```python
from build123d import *

# Parameters (mm, degrees)
BOSS_EXTRUDE1_DEPTH = 55
SKETCH2_W           = 12
SKETCH2_H           = 4.5
SKETCH2_W_2         = 11.8
SKETCH2_H_2         = 4.3
BOSS_EXTRUDE2_DEPTH = 12.5
SKETCH3_W           = 11.8
SKETCH3_H           = 1.5
BOSS_EXTRUDE3_DEPTH = 12.4
CUT_EXTRUDE1_DEPTH  = 0.5
SKETCH6_W           = 10.75
SKETCH6_H           = 9
CUT_EXTRUDE2_DEPTH  = 3
SKETCH7_W           = 5.5
SKETCH7_H           = 2.3
BOSS_EXTRUDE4_DEPTH = 0.1
SKETCH8_R           = 0.3
BOSS_EXTRUDE5_DEPTH = 6
LPATTERN1_COUNT     = 3
LPATTERN1_PITCH     = 2.9
SKETCH9_W           = 15.5
SKETCH9_H           = 3.5
CUT_EXTRUDE3_DEPTH  = 2
SKETCH10_R          = 0.3
BOSS_EXTRUDE6_DEPTH = 6
LPATTERN2_COUNT     = 6
LPATTERN2_PITCH     = 2.5
FILLET1_R           = 1.25


with BuildPart() as part:
    # Sketch1 → Boss-Extrude1 (new body)
    with BuildSketch(Plane.XY):
        Polygon((-12.5, 0), (-12, -6.2), (12, -6.2), (12.5, 0), (12.5, 5.5), (-12.5, 5.5), align=None)
    extrude(amount=-BOSS_EXTRUDE1_DEPTH)

    # Sketch2 → Boss-Extrude2 (add)
    with BuildSketch(Plane.XY):
        Rectangle(SKETCH2_W, SKETCH2_H)
        Rectangle(SKETCH2_W_2, SKETCH2_H_2, mode=Mode.SUBTRACT)
    extrude(amount=BOSS_EXTRUDE2_DEPTH)

    # Sketch3 → Boss-Extrude3 (add)
    with BuildSketch(Plane.XY):
        with Locations((0, -1.4)):
            Rectangle(SKETCH3_W, SKETCH3_H)
    extrude(amount=BOSS_EXTRUDE3_DEPTH)

    # Sketch4 → Cut-Extrude1 (cut)
    with BuildSketch(Plane(origin=(0, 2.25, 0), x_dir=(1, 0, 0), z_dir=(0, 1, 0))):
        with BuildLine():
            Line((-4.25, -5.3), (-1.95, -5.3))
            ThreePointArc((-1.95, -5.3), (-1.808578644, -5.358578644), (-1.75, -5.5))
            Line((-1.75, -5.5), (-1.75, -7.3))
            ThreePointArc((-1.75, -7.3), (-1.808578644, -7.441421356), (-1.95, -7.5))
            Line((-1.95, -7.5), (-4.25, -7.5))
            ThreePointArc((-4.25, -7.5), (-4.391421356, -7.441421356), (-4.45, -7.3))
            Line((-4.45, -7.3), (-4.45, -5.5))
            ThreePointArc((-4.45, -5.5), (-4.391421356, -5.358578644), (-4.25, -5.3))
        make_face()
        with BuildLine():
            Line((1.95, -5.3), (4.25, -5.3))
            ThreePointArc((4.25, -5.3), (4.391421356, -5.358578644), (4.45, -5.5))
            Line((4.45, -5.5), (4.45, -7.3))
            ThreePointArc((4.45, -7.3), (4.391421356, -7.441421356), (4.25, -7.5))
            Line((4.25, -7.5), (1.95, -7.5))
            ThreePointArc((1.95, -7.5), (1.808578644, -7.441421356), (1.75, -7.3))
            Line((1.75, -7.3), (1.75, -5.5))
            ThreePointArc((1.75, -5.5), (1.808578644, -5.358578644), (1.95, -5.3))
        make_face()
    extrude(amount=-CUT_EXTRUDE1_DEPTH, mode=Mode.SUBTRACT)

    # Sketch6 → Cut-Extrude2 (cut)
    with BuildSketch(Plane(origin=(0, 5.5, 0), x_dir=(1, 0, 0), z_dir=(0, 1, 0))):
        with Locations((-7.125, 18)):
            Rectangle(SKETCH6_W, SKETCH6_H)
    extrude(amount=-CUT_EXTRUDE2_DEPTH, mode=Mode.SUBTRACT)

    # Sketch7 → Boss-Extrude4 (add)
    with BuildSketch(Plane(origin=(0, 2.5, 0), x_dir=(1, 0, 0), z_dir=(0, 1, 0))):
        with Locations((-6.75, 15.15)):
            Rectangle(SKETCH7_W, SKETCH7_H)
    boss_extrude4 = extrude(amount=BOSS_EXTRUDE4_DEPTH)

    # Sketch8 → Boss-Extrude5 (add)
    with BuildSketch(Plane(origin=(0, 2.6, 0), x_dir=(1, 0, 0), z_dir=(0, 1, 0))):
        with Locations(Location((-8, 15.15, 0), (0, 0, 180))):
            Circle(SKETCH8_R)
        with Locations(Location((-5.5, 15.15, 0), (0, 0, 180))):
            Circle(SKETCH8_R)
    boss_extrude5 = extrude(amount=BOSS_EXTRUDE5_DEPTH)

    # LPattern1: Boss-Extrude4, Boss-Extrude5 ×3
    with Locations(*[(0, 0, -i * LPATTERN1_PITCH) for i in range(1, LPATTERN1_COUNT)]):
        add(boss_extrude4)
        add(boss_extrude5)

    # Sketch9 → Cut-Extrude3 (cut)
    with BuildSketch(Plane(origin=(0, 0, -55), x_dir=(-1, 0, 0), z_dir=(0, 0, -1))):
        with Locations((0, 1.75)):
            Rectangle(SKETCH9_W, SKETCH9_H)
    extrude(amount=-CUT_EXTRUDE3_DEPTH, mode=Mode.SUBTRACT)

    # Sketch10 → Boss-Extrude6 (add)
    with BuildSketch(Plane(origin=(0, 0, -53), x_dir=(-1, 0, 0), z_dir=(0, 0, -1))):
        with Locations((-6.25, 1.75)):
            Circle(SKETCH10_R)
    boss_extrude6 = extrude(amount=BOSS_EXTRUDE6_DEPTH)

    # LPattern2: Boss-Extrude6 ×6
    with Locations(*[(-i * LPATTERN2_PITCH, 0, 0) for i in range(1, LPATTERN2_COUNT)]):
        add(boss_extrude6)

    # Fillet1
    # the kernel refuses this fillet: 1.25 mm, written as the material it takes off along each edge
    with BuildSketch(Plane(origin=(11.25, 4.25, -1.25), x_dir=(0, 0, 1), z_dir=(1, 0, 0))) as fillet1_piece_1_section:
        Polygon((0, 0), (FILLET1_R * 1.02, 0), (FILLET1_R * 1.02, -FILLET1_R * 1.02), (0, -FILLET1_R * 1.02), align=None)
    fillet1_piece_1 = extrude(amount=FILLET1_R * 1.02, mode=Mode.PRIVATE)
    fillet1_piece_1 = fillet1_piece_1 - Plane(origin=(11.25, 4.25, -1.25), x_dir=(0, -0.7071067811865475, -0.7071067811865475), z_dir=(1, 0, 0)) * Sphere(FILLET1_R, mode=Mode.PRIVATE)
    add(fillet1_piece_1, mode=Mode.SUBTRACT)
    with BuildSketch(Plane(origin=(-11.25, 4.25, -1.25), x_dir=(0, 0, 1), z_dir=(-1, 0, 0))) as fillet1_piece_2_section:
        Polygon((0, 0), (FILLET1_R * 1.02, 0), (FILLET1_R * 1.02, FILLET1_R * 1.02), (0, FILLET1_R * 1.02), align=None)
    fillet1_piece_2 = extrude(amount=FILLET1_R * 1.02, mode=Mode.PRIVATE)
    fillet1_piece_2 = fillet1_piece_2 - Plane(origin=(-11.25, 4.25, -1.25), x_dir=(0, -0.7071067811865475, -0.7071067811865475), z_dir=(-1, 0, 0)) * Sphere(FILLET1_R, mode=Mode.PRIVATE)
    add(fillet1_piece_2, mode=Mode.SUBTRACT)
    with BuildSketch(Plane(origin=(-11.25, 4.25, -53.75), x_dir=(0, 0, -1), z_dir=(-1, 0, 0))) as fillet1_piece_3_section:
        Polygon((0, 0), (FILLET1_R * 1.02, 0), (FILLET1_R * 1.02, -FILLET1_R * 1.02), (0, -FILLET1_R * 1.02), align=None)
    fillet1_piece_3 = extrude(amount=FILLET1_R * 1.02, mode=Mode.PRIVATE)
    fillet1_piece_3 = fillet1_piece_3 - Plane(origin=(-11.25, 4.25, -53.75), x_dir=(0, -0.7071067811865475, 0.7071067811865475), z_dir=(-1, 0, 0)) * Sphere(FILLET1_R, mode=Mode.PRIVATE)
    add(fillet1_piece_3, mode=Mode.SUBTRACT)
    with BuildSketch(Plane(origin=(11.25, 4.25, -53.75), x_dir=(0, 0, -1), z_dir=(1, 0, 0))) as fillet1_piece_4_section:
        Polygon((0, 0), (FILLET1_R * 1.02, 0), (FILLET1_R * 1.02, FILLET1_R * 1.02), (0, FILLET1_R * 1.02), align=None)
    fillet1_piece_4 = extrude(amount=FILLET1_R * 1.02, mode=Mode.PRIVATE)
    fillet1_piece_4 = fillet1_piece_4 - Plane(origin=(11.25, 4.25, -53.75), x_dir=(0, -0.7071067811865475, 0.7071067811865475), z_dir=(1, 0, 0)) * Sphere(FILLET1_R, mode=Mode.PRIVATE)
    add(fillet1_piece_4, mode=Mode.SUBTRACT)
    with BuildSketch(Plane(origin=(-19.5, -6.2, 0), x_dir=(0, 0, -1), z_dir=(1, 0, 0))) as fillet1_piece_5:
        with BuildLine():
            CenterArc((FILLET1_R, FILLET1_R), FILLET1_R, 180, 90)
            Line((0, FILLET1_R), (-FILLET1_R * 0.02, FILLET1_R))
            Line((-FILLET1_R * 0.02, FILLET1_R), (-FILLET1_R * 0.02, -FILLET1_R * 0.02))
            Line((-FILLET1_R * 0.02, -FILLET1_R * 0.02), (FILLET1_R, -FILLET1_R * 0.02))
            Line((FILLET1_R, -FILLET1_R * 0.02), (FILLET1_R, 0))
        make_face()
    extrude(amount=39, mode=Mode.SUBTRACT)
    with BuildSketch(Plane(origin=(11.25, 5.5, 0), x_dir=(0, -1, 0), z_dir=(-1, 0, 0))) as fillet1_piece_6:
        with BuildLine():
            CenterArc((FILLET1_R, -FILLET1_R), FILLET1_R, 90, 90)
            Line((0, -FILLET1_R), (-FILLET1_R * 0.02, -FILLET1_R))
            Line((-FILLET1_R * 0.02, -FILLET1_R), (-FILLET1_R * 0.02, FILLET1_R * 0.02))
            Line((-FILLET1_R * 0.02, FILLET1_R * 0.02), (FILLET1_R, FILLET1_R * 0.02))
            Line((FILLET1_R, FILLET1_R * 0.02), (FILLET1_R, 0))
        make_face()
    extrude(amount=22.5, mode=Mode.SUBTRACT)
    with BuildSketch(Plane(origin=(-12.5, 5.5, -1.25), x_dir=(0, -1, 0), z_dir=(0, 0, -1))) as fillet1_piece_7:
        with BuildLine():
            CenterArc((FILLET1_R, -FILLET1_R), FILLET1_R, 90, 90)
            Line((0, -FILLET1_R), (-FILLET1_R * 0.02, -FILLET1_R))
            Line((-FILLET1_R * 0.02, -FILLET1_R), (-FILLET1_R * 0.02, FILLET1_R * 0.02))
            Line((-FILLET1_R * 0.02, FILLET1_R * 0.02), (FILLET1_R, FILLET1_R * 0.02))
            Line((FILLET1_R, FILLET1_R * 0.02), (FILLET1_R, 0))
        make_face()
    extrude(amount=19.75, mode=Mode.SUBTRACT)
    with BuildSketch(Plane(origin=(-12.5, 5.5, -15), x_dir=(0, -1, 0), z_dir=(0, 0, -1))) as fillet1_piece_8:
        with BuildLine():
            CenterArc((FILLET1_R, -FILLET1_R), FILLET1_R, 90, 90)
            Line((0, -FILLET1_R), (-FILLET1_R * 0.02, -FILLET1_R))
            Line((-FILLET1_R * 0.02, -FILLET1_R), (-FILLET1_R * 0.02, FILLET1_R * 0.02))
            Line((-FILLET1_R * 0.02, FILLET1_R * 0.02), (FILLET1_R, FILLET1_R * 0.02))
            Line((FILLET1_R, FILLET1_R * 0.02), (FILLET1_R, 0))
        make_face()
    extrude(amount=38.75, mode=Mode.SUBTRACT)
    with BuildSketch(Plane(origin=(-12, -6.2, 6.919510423), x_dir=(-0.08038418992031013, 0.9967639550118451, 0), z_dir=(0, 0, -1)), Plane(origin=(12, -6.2, 6.919510423), x_dir=(-1, 0, 0), z_dir=(0, 0, -1))) as fillet1_piece_9:
        with BuildLine():
            CenterArc((FILLET1_R * 0.922601389683, FILLET1_R), FILLET1_R, 184.610649319, 85.389350681)
            Line((-FILLET1_R * 0.074162565329, FILLET1_R * 0.91961581008), (-FILLET1_R * 0.0940978444292, FILLET1_R * 0.918008126281))
            Line((-FILLET1_R * 0.0940978444292, FILLET1_R * 0.918008126281), (-FILLET1_R * 0.0184520277937, -FILLET1_R * 0.02))
            Line((-FILLET1_R * 0.0184520277937, -FILLET1_R * 0.02), (FILLET1_R * 0.922601389683, -FILLET1_R * 0.02))
            Line((FILLET1_R * 0.922601389683, -FILLET1_R * 0.02), (FILLET1_R * 0.922601389683, 0))
        make_face()
    extrude(amount=68.839020845, mode=Mode.SUBTRACT)
    with BuildSketch(Plane(origin=(-19.5, -6.2, -55), x_dir=(0, 0, 1), z_dir=(1, 0, 0))) as fillet1_piece_10:
        with BuildLine():
            CenterArc((FILLET1_R, -FILLET1_R), FILLET1_R, 90, 90)
            Line((0, -FILLET1_R), (-FILLET1_R * 0.02, -FILLET1_R))
            Line((-FILLET1_R * 0.02, -FILLET1_R), (-FILLET1_R * 0.02, FILLET1_R * 0.02))
            Line((-FILLET1_R * 0.02, FILLET1_R * 0.02), (FILLET1_R, FILLET1_R * 0.02))
            Line((FILLET1_R, FILLET1_R * 0.02), (FILLET1_R, 0))
        make_face()
    extrude(amount=39, mode=Mode.SUBTRACT)
    with BuildSketch(Plane(origin=(11.25, 5.5, -55), x_dir=(0, -1, 0), z_dir=(-1, 0, 0))) as fillet1_piece_11:
        with BuildLine():
            CenterArc((FILLET1_R, FILLET1_R), FILLET1_R, 180, 90)
            Line((0, FILLET1_R), (-FILLET1_R * 0.02, FILLET1_R))
            Line((-FILLET1_R * 0.02, FILLET1_R), (-FILLET1_R * 0.02, -FILLET1_R * 0.02))
            Line((-FILLET1_R * 0.02, -FILLET1_R * 0.02), (FILLET1_R, -FILLET1_R * 0.02))
            Line((FILLET1_R, -FILLET1_R * 0.02), (FILLET1_R, 0))
        make_face()
    extrude(amount=22.5, mode=Mode.SUBTRACT)
    with BuildSketch(Plane(origin=(12.5, 5.5, -1.25), x_dir=(-1, 0, 0), z_dir=(0, 0, -1))) as fillet1_piece_12:
        with BuildLine():
            CenterArc((FILLET1_R, -FILLET1_R), FILLET1_R, 90, 90)
            Line((0, -FILLET1_R), (-FILLET1_R * 0.02, -FILLET1_R))
            Line((-FILLET1_R * 0.02, -FILLET1_R), (-FILLET1_R * 0.02, FILLET1_R * 0.02))
            Line((-FILLET1_R * 0.02, FILLET1_R * 0.02), (FILLET1_R, FILLET1_R * 0.02))
            Line((FILLET1_R, FILLET1_R * 0.02), (FILLET1_R, 0))
        make_face()
    extrude(amount=52.5, mode=Mode.SUBTRACT)
    with BuildSketch(Plane(origin=(12.5, -7.5, -55), x_dir=(-1, 0, 0), z_dir=(0, 1, 0)), Plane(origin=(-12.5, 4.25, 0), x_dir=(0, 0, -1), z_dir=(0, -1, 0))) as fillet1_piece_13:
        with BuildLine():
            CenterArc((FILLET1_R, FILLET1_R), FILLET1_R, 180, 90)
            Line((0, FILLET1_R), (-FILLET1_R * 0.02, FILLET1_R))
            Line((-FILLET1_R * 0.02, FILLET1_R), (-FILLET1_R * 0.02, -FILLET1_R * 0.02))
            Line((-FILLET1_R * 0.02, -FILLET1_R * 0.02), (FILLET1_R, -FILLET1_R * 0.02))
            Line((FILLET1_R, -FILLET1_R * 0.02), (FILLET1_R, 0))
        make_face()
    extrude(amount=11.75, mode=Mode.SUBTRACT)
    with BuildSketch(Plane(origin=(-12.5, 4.25, -55), x_dir=(0, 0, 1), z_dir=(0, -1, 0)), Plane(origin=(12.5, -7.5, 0), x_dir=(-1, 0, 0), z_dir=(0, 1, 0))) as fillet1_piece_14:
        with BuildLine():
            CenterArc((FILLET1_R, -FILLET1_R), FILLET1_R, 90, 90)
            Line((0, -FILLET1_R), (-FILLET1_R * 0.02, -FILLET1_R))
            Line((-FILLET1_R * 0.02, -FILLET1_R), (-FILLET1_R * 0.02, FILLET1_R * 0.02))
            Line((-FILLET1_R * 0.02, FILLET1_R * 0.02), (FILLET1_R, FILLET1_R * 0.02))
            Line((FILLET1_R, FILLET1_R * 0.02), (FILLET1_R, 0))
        make_face()
    extrude(amount=11.75, mode=Mode.SUBTRACT)


solid = part.part
```
Input: part model. Units: mm. Frame: model coordinates. A direction names the side the tool comes from. Give positions to 0.01 mm unless a question says otherwise; leave off trailing zeros. Order: outer loops, then holes, each group sorted by start corner. A loop starts at its lowest first (then second) coordinate and runs counter-clockwise, first axis right, second up. Notation, with made-up numbers: M -9,-1 L 14,-1 A12 cw 14,6 Z; hole C 3.25,87 d7. An arc over 180 degrees is marked long. One line per question, with ' | ' between items. Start each with the question number.
1. Section query B-B (y = -3.75). Return the cut outline in (x, z).
2. Section query A-A (z = -34.5). Return the cut outline in (x, y).
3. Access query for faces 4 (the face through (0, 3.5, -54)), 5 (the face through (-6, -1, 6)), 6 (the face through (0, -2.25, 6)), 7 (the face through (-7, 2.6, -18)). Directions: +Z, -Z, +X, -X, +Y, -Y. A direction counts if a zero-diameter tool reaches every point of the face in a straight line with its end or side. Return the directions, or none.
4. Pull-direction query (Z, two-part tool) for faces 1 (the face through (11.96, 0.35, -0.22)), 2 (the face through (-11.68, -5.88, -27.12)), 3 (the face through (-7, 4, -13.5)); classes: released by +Z, released by -Z, zero draft, split by the parting line, or undercut.
5. Material intervals for probe 1 along Y at (x, z) = (-1.5, -5.5); probe 2 along Z at (x, y) = (-6.25, -0.75); probe 3 along Y at (x, z) = (6.25, -54), sorted ascending. Write a range as [from, to].
6. First-contact query: pin 1 Ø1.3 at (y, z) = (0, 5.5) entering from -X; pin 2 Ø1 at (x, y) = (1, -1) entering from +Z; pin 3 Ø0.7 at (x, z) = (-6.5, -20.5) entering from +Y. Flat tips, straight axial feed; report the tip coordinate or a pass-through.
Here are the results:
1) outline: M -12.2,-54.57 A1.25 ccw -11.25,-55 L 11.25,-55 A1.25 ccw 12.2,-54.57 L 12.2,-0.43 A1.25 ccw 11.25,0 L -11.25,0 A1.25 ccw -12.2,-0.43 Z
2) outline: M -12.5,0 L -12.09,-5.05 A1.25 ccw -10.85,-6.2 L 10.85,-6.2 A1.25 ccw 12.09,-5.05 L 12.5,0 L 12.5,4.25 A1.25 ccw 11.25,5.5 L -11.25,5.5 A1.25 ccw -12.5,4.25 Z
3) face 4: -Z | face 5: +Z, -X, +Y, -Y | face 6: +Z, +X, -X, -Y | face 7: +Y
4) face 1: released by +Z | face 2: zero draft | face 3: undercut
5) probe 1: [-6.2, 5.5] | probe 2: [-55, 0] | probe 3: [-6.17, 0], [1.45, 2.05], [3.5, 5.47]
6) pin 1: x = -6 | pin 2: z = 12.4 | pin 3: y = 2.6
